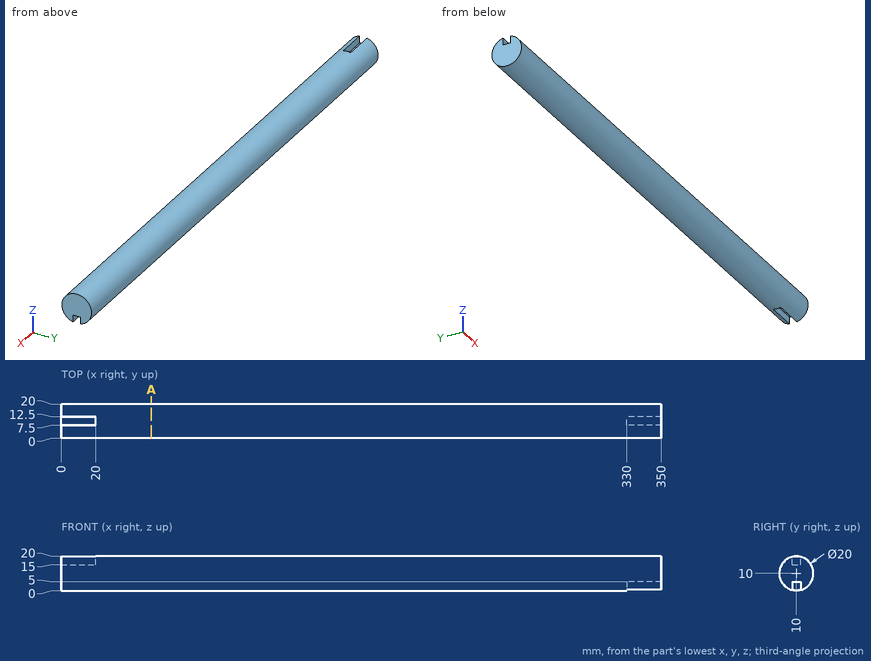
Verification items for this drawing (mm, ordinates from the low corner). Coordinates: 2 decimals unless noted, no trailing zeros. Loops run counter-clockwise (first coordinate to the right, second up) from the corner with the lowest first, then second, coordinate; pieces in that order, holes last. Notation, with made-up numbers: (26, 81.5) -> (53, 81.5) arc R9 ccw to (53, 86.5) -> close; hole circle Ø9 at (-21.75, 11). An arc over 180 degrees is marked (long way). Put each result on its own line as item: value.
1. Gauge pin test, flat ends, axial feed: P1, Ø5, axis at x = 214.5, z = 5, coming from the +Y side; P2, Ø1.5, axis at x = 7.5, y = 9.5, coming from the +Z side; P3, Ø3, axis at x = 225, y = 16, coming from the -Z side; P4, Ø8, axis at y = 8.5, z = 7.5, coming from the -X side. Record the tip position at first contact, or that the pin passes through.
Result set:
P1: stops at y = 19.68
P2: stops at z = 15
P3: stops at z = 1.07
P4: stops at x = 0
2. Thickness scan on line 1 (Z direction, x = 317.5, y = 12.75); line 2 (Y direction, x = 124, z = 6.25). Record the ranges inside material, lowest first.
Result set:
line 1: z = 0.39 to 19.61
line 2: y = 0.73 to 19.27
3. Section check A-A, the plane x = 52.5. Record the boundary of the cut face in (y, z).
Result set:
outline: circle Ø20 at (10, 10)
